Geometry check sheet. Reference: the model listing, model coordinates, mm. Face numbers are marked on the shaded views. A direction names the side the tool comes from. Round coordinates to 2 decimals unless told otherwise and drop trailing zeros. Order: outer loops, then holes, each group sorted by start corner. A loop starts at its lowest first (then second) coordinate and runs counter-clockwise, first axis right, second up. Notation, with made-up numbers: (34.25, 14) - (58.25, 14) arc R31 ccw to (58.25, 53) - close; hole circle Ø6 at (45, 2). An arc over 180 degrees is marked (long way). Use a Markdown table: item, result. Add a question column.
(1) Mould release check, pull along Z, two halves, no side actions. Record for the marked faces 4, 5 and 6: released by +Z, released by -Z, zero draft, split by the parting line, or undercut.
(2) Thickness scan on line 1 along X through (y, z) = (15.5, -7.1); line 2 along Y through (x, z) = (15.5, -4.4). Record the ranges inside material, lowest first. Write a range as [from, to].
(3) Access from +Z, -Z, +X, -X, +Y, -Y to the whole of each face (thin tool, end or side, straight path). Record for the marked faces 1, 2 and 3.
(4) Section check C-C on z = -11.5. Record the boundary of the cut face in (x, y).
(5) Section check A-A on y = 0. Record the boundary of the cut face in (x, z), then the cut area to 3 significant figures.
(6) Gauge pin test, flat ends, axial feed: P1, Ø2, axis at x = -15.5, y = -15.5, coming from the +Z side; P2, Ø4, axis at x = 5.5, z = -14, coming from the -Y side; P3, Ø0.5, axis at x = -0.5, y = 2.5, coming from the +Z side. Record the tip position at first contact, or that the pin passes through.
(7) Section check D-D on x = -5. Record the boundary of the cut face in (y, z).
(8) Section check B-B on x = -12. Record the boundary of the cut face in (y, z), then the cut area to 3 significant figures.
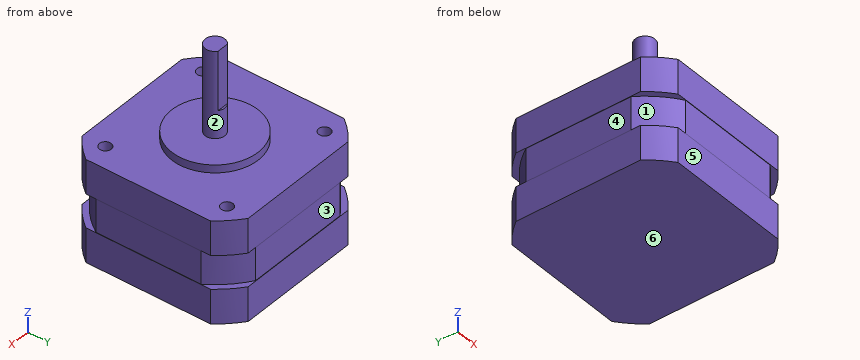
```python
from build123d import *

# Parameters (mm, degrees)
SKETCH1_R                       = 2.5
BOSS_EXTRUDE1_DEPTH             = 24
SKETCH2_R                       = 11
BOSS_EXTRUDE2_DEPTH             = 2
SKETCH3_W                       = 42.418
SKETCH3_H                       = 42.418
BOSS_EXTRUDE3_DEPTH             = 26
CUT_EXTRUDE1_DEPTH              = 59.306460723
M3X0_5_TAPPED_HOLE1_D           = 2.5
M3X0_5_TAPPED_HOLE1_DEPTH       = 7.5
M3X0_5_TAPPED_HOLE1_CBORE_D     = 3
M3X0_5_TAPPED_HOLE1_CBORE_DEPTH = 6
M3X0_5_TAPPED_HOLE1_TIP         = 0.751075774
CUT_EXTRUDE2_START              = -15
CUT_EXTRUDE2_DEPTH              = 15
CUT_EXTRUDE3_DEPTH              = 4.25
CUT_EXTRUDE3_DEPTH_BACK         = 4.25


with BuildPart() as part:
    # Sketch1 → Boss-Extrude1 (new body)
    with BuildSketch(Plane.XY):
        Circle(SKETCH1_R)
    extrude(amount=BOSS_EXTRUDE1_DEPTH)

    # Sketch2 → Boss-Extrude2 (add)
    with BuildSketch(Plane(origin=(0, 0, 0), x_dir=(-1, 0, 0), z_dir=(0, 0, -1))):
        Circle(SKETCH2_R)
    extrude(amount=-BOSS_EXTRUDE2_DEPTH)

    # Sketch3 → Boss-Extrude3 (add)
    with BuildSketch(Plane(origin=(0, 0, 0), x_dir=(-1, 0, 0), z_dir=(0, 0, -1))):
        Rectangle(SKETCH3_W, SKETCH3_H)
    extrude(amount=BOSS_EXTRUDE3_DEPTH)

    # Sketch4 → Cut-Extrude1 (cut, through all)
    with BuildSketch(Plane(origin=(0, 0, -26), x_dir=(-1, 0, 0), z_dir=(0, 0, -1))):
        with BuildLine():
            Line((-21.209, -15.887992919), (-21.209, -21.209))
            Line((-21.209, -21.209), (-15.887992919, -21.209))
            ThreePointArc((-15.887992919, -21.209), (-18.738329701, -18.738329701), (-21.209, -15.887992919))
        make_face()
        with BuildLine():
            Line((15.887992919, -21.209), (21.209, -21.209))
            Line((21.209, -21.209), (21.209, -15.887992919))
            ThreePointArc((21.209, -15.887992919), (18.738329701, -18.738329701), (15.887992919, -21.209))
        make_face()
        with BuildLine():
            Line((21.209, 15.887992919), (21.209, 21.209))
            Line((21.209, 21.209), (15.887992919, 21.209))
            ThreePointArc((15.887992919, 21.209), (18.738329701, 18.738329701), (21.209, 15.887992919))
        make_face()
        with BuildLine():
            Line((-15.887992919, 21.209), (-21.209, 21.209))
            Line((-21.209, 21.209), (-21.209, 15.887992919))
            ThreePointArc((-21.209, 15.887992919), (-18.738329701, 18.738329701), (-15.887992919, 21.209))
        make_face()
    extrude(amount=-CUT_EXTRUDE1_DEPTH, mode=Mode.SUBTRACT)

    # M3x0.5 Tapped Hole1
    with Locations(Plane.XY):
        with Locations((-15.5, 15.5), (-15.5, -15.5), (15.5, -15.5), (15.5, 15.5)):
            CounterBoreHole(M3X0_5_TAPPED_HOLE1_D / 2, M3X0_5_TAPPED_HOLE1_CBORE_D / 2, M3X0_5_TAPPED_HOLE1_CBORE_DEPTH, depth=M3X0_5_TAPPED_HOLE1_DEPTH)
            with Locations((0, 0, -(M3X0_5_TAPPED_HOLE1_DEPTH + M3X0_5_TAPPED_HOLE1_TIP / 2))):  # 118° drill point
                Cone(0, M3X0_5_TAPPED_HOLE1_D / 2, M3X0_5_TAPPED_HOLE1_TIP, mode=Mode.SUBTRACT)

    # Sketch7 → Cut-Extrude2 (cut)
    with BuildSketch(Plane.XY.offset(24).offset(CUT_EXTRUDE2_START)):
        with BuildLine():
            Line((-1.5, 2), (1.5, 2))
            ThreePointArc((1.5, 2), (0, 2.5), (-1.5, 2))
        make_face()
    extrude(amount=CUT_EXTRUDE2_DEPTH, mode=Mode.SUBTRACT)

    # Sketch8 → Cut-Extrude3 (cut, two sides: drawn at the far end of the back side and taken through both)
    with BuildSketch(Plane.XY.offset(-13).offset(-CUT_EXTRUDE3_DEPTH_BACK)):
        with BuildLine():
            Line((15.887992919, 21.209), (-15.887992919, 21.209))
            ThreePointArc((-15.887992919, 21.209), (-18.738329701, 18.738329701), (-21.209, 15.887992919))
            Line((-21.209, 15.887992919), (-21.209, -15.887992919))
            ThreePointArc((-21.209, -15.887992919), (-18.738329701, -18.738329701), (-15.887992919, -21.209))
            Line((-15.887992919, -21.209), (15.887992919, -21.209))
            ThreePointArc((15.887992919, -21.209), (18.738329701, -18.738329701), (21.209, -15.887992919))
            Line((21.209, -15.887992919), (21.209, 15.887992919))
            ThreePointArc((21.209, 15.887992919), (18.738329701, 18.738329701), (15.887992919, 21.209))
        make_face()
        with BuildLine():
            Line((-13.394406258, 21.109), (13.394406258, 21.109))
            ThreePointArc((13.394406258, 21.109), (17.67766953, 17.67766953), (21.109, 13.394406258))
            Line((21.109, 13.394406258), (21.109, -13.394406258))
            ThreePointArc((21.109, -13.394406258), (17.67766953, -17.67766953), (13.394406258, -21.109))
            Line((13.394406258, -21.109), (-13.394406258, -21.109))
            ThreePointArc((-13.394406258, -21.109), (-17.67766953, -17.67766953), (-21.109, -13.394406258))
            Line((-21.109, -13.394406258), (-21.109, 13.394406258))
            ThreePointArc((-21.109, 13.394406258), (-17.67766953, 17.67766953), (-13.394406258, 21.109))
        make_face(mode=Mode.SUBTRACT)
    extrude(amount=CUT_EXTRUDE3_DEPTH + CUT_EXTRUDE3_DEPTH_BACK, mode=Mode.SUBTRACT)


solid = part.part
```
Check sheet entries:
| question | item | result |
|---|---|---|
| 1 | face 4 | undercut |
| 1 | face 5 | zero draft |
| 1 | face 6 | released by -Z |
| 2 | line 1 | x = [-21.21, -16.75], [-14.25, 14.25], [16.75, 21.21] |
| 2 | line 2 | y = [-21.21, -17], [-14, 14], [17, 21.21] |
| 3 | face 1 | -X, -Y |
| 3 | face 2 | +Z |
| 3 | face 3 | +X, -X, +Y |
| 4 | outline | (-21.11, -13.39) arc R25 ccw to (-13.39, -21.11) - (13.39, -21.11) arc R25 ccw to (21.11, -13.39) - (21.11, 13.39) arc R25 ccw to (13.39, 21.11) - (-13.39, 21.11) arc R25 ccw to (-21.11, 13.39) - close |
| 5 | outline | (-21.21, -26) - (21.21, -26) - (21.21, -17.25) - (21.11, -17.25) - (21.11, -8.75) - (21.21, -8.75) - (21.21, 0) - (11, 0) - (11, 2) - (2.5, 2) - (2.5, 24) - (-2.5, 24) - (-2.5, 2) - (-11, 2) - (-11, 0) - (-21.21, 0) - (-21.21, -8.75) - (-21.11, -8.75) - (-21.11, -17.25) - (-21.21, -17.25) - close |
| 5 | area | 1,260 mm2 |
| 6 | P1 | stops at z = -7.65 |
| 6 | P2 | stops at y = -21.11 |
| 6 | P3 | stops at z = 9 |
| 7 | outline | (-21.21, -26) - (21.21, -26) - (21.21, -17.25) - (21.11, -17.25) - (21.11, -8.75) - (21.21, -8.75) - (21.21, 0) - (9.8, 0) - (9.8, 2) - (-9.8, 2) - (-9.8, 0) - (-21.21, 0) - (-21.21, -8.75) - (-21.11, -8.75) - (-21.11, -17.25) - (-21.21, -17.25) - close |
| 8 | outline | (-21.21, -26) - (21.21, -26) - (21.21, -17.25) - (21.11, -17.25) - (21.11, -8.75) - (21.21, -8.75) - (21.21, 0) - (-21.21, 0) - (-21.21, -8.75) - (-21.11, -8.75) - (-21.11, -17.25) - (-21.21, -17.25) - close |
| 8 | area | 1,100 mm2 |
